```python
from build123d import *

# Parameters (mm, degrees)
SKETCH2_W           = 457.2
SKETCH2_H           = 457.2
BOSS_EXTRUDE3_DEPTH = 4.445
SKETCH3_R           = 3.175
SKETCH3_R_2         = 3.9751
CUT_EXTRUDE1_DEPTH  = 324.31977673
SKETCH4_W           = 457.2
SKETCH4_H           = 457.2
SKETCH4_R           = 3.175
CUT_EXTRUDE2_DEPTH  = 324.31977673


with BuildPart() as part:
    # Sketch2 → Boss-Extrude3 (new body)
    with BuildSketch(Plane.XY):
        Rectangle(SKETCH2_W, SKETCH2_H)
    extrude(amount=BOSS_EXTRUDE3_DEPTH)

    # Sketch3 → Cut-Extrude1 (cut, through all)
    with BuildSketch(Plane(origin=(0, 0, 0), x_dir=(-1, 0, 0), z_dir=(0, 0, -1))):
        with Locations((-138.143199548, 71.871365193)):
            Circle(SKETCH3_R)
        with Locations((-198.809547248, -25.000118004)):
            Circle(SKETCH3_R)
        with Locations((-122.004659563, -96.265887155)):
            Circle(SKETCH3_R)
        with Locations((-26.754659563, -96.265887155)):
            Circle(SKETCH3_R)
        with Locations((-26.754659563, 23.469712845)):
            Circle(SKETCH3_R_2)
    extrude(amount=-CUT_EXTRUDE1_DEPTH, mode=Mode.SUBTRACT)

    # Sketch4 → Cut-Extrude2 (cut, through all)
    # profile 1 of 5: a face of its own
    with BuildSketch(Plane.XY.offset(4.445)):
        Rectangle(SKETCH4_W, SKETCH4_H)
        with Locations((26.754659563, -96.265887155)):
            Circle(SKETCH4_R, mode=Mode.SUBTRACT)
        with BuildLine():
            Line((104.279919091, -89.284764381), (29.57120013, 4.629075933))
            ThreePointArc((29.57120013, 4.629075933), (8.270979184, 28.080142289), (38.089671454, 38.780493538))
            Line((38.089671454, 38.780493538), (119.216168571, 74.032383096))
            ThreePointArc((119.216168571, 74.032383096), (139.225456422, 90.890598092), (157.193199548, 71.871365193))
            ThreePointArc((157.193199548, 71.871365193), (156.629627395, 67.271964637), (154.972256192, 62.944699943))
            Line((154.972256192, 62.944699943), (198.125737804, -5.962394804))
            ThreePointArc((198.125737804, -5.962394804), (212.035958895, -11.290102141), (217.859547248, -25.000118004))
            ThreePointArc((217.859547248, -25.000118004), (210.121888692, -40.327656327), (193.194620104, -43.203828976))
            Line((193.194620104, -43.203828976), (140.576999281, -92.026701216))
            ThreePointArc((140.576999281, -92.026701216), (140.934867851, -94.13288125), (141.054659563, -96.265887155))
            ThreePointArc((141.054659563, -96.265887155), (118.451759762, -114.981639959), (104.279919091, -89.284764381))
        make_face(mode=Mode.SUBTRACT)
    # profile 2 of 5: a face of its own
    with BuildSketch(Plane.XY.offset(4.445)):
        with BuildLine():
            ThreePointArc((127.085491453, 56.359125133), (126.946386449, 56.459231128), (126.808187657, 56.5605845))
            Line((126.808187657, 56.5605845), (55.070704112, 25.388502171))
            Line((55.070704112, 25.388502171), (122.29505865, 6.450632186))
            Line((122.29505865, 6.450632186), (127.085491453, 56.359125133))
        make_face()
    # profile 3 of 5: a face of its own
    with BuildSketch(Plane.XY.offset(4.445)):
        Polygon((144.946705866, 43.06176458), (140.928758156, 1.201305791), (177.638536292, -9.140258814), align=None)
    # profile 4 of 5: a face of its own
    with BuildSketch(Plane.XY.offset(4.445)):
        Polygon((179.886249099, -29.564951481), (139.079100318, -18.069110674), (133.87810257, -72.255020413), align=None)
    # profile 5 of 5: a face of its own
    with BuildSketch(Plane.XY.offset(4.445)):
        Polygon((120.445400812, -12.81978428), (52.587094953, 6.296677047), (114.776579601, -71.879651121), align=None)
    extrude(amount=-CUT_EXTRUDE2_DEPTH, mode=Mode.SUBTRACT)


solid = part.part
```
Verification items for the finished model (mm, model axes). A direction names the side the tool comes from. Round coordinates to 2 decimals unless told otherwise and drop trailing zeros. Write each loop counter-clockwise with the first axis right and the second up, starting at its lowest first coordinate (ties: lowest second). Pieces come first, ordered by that corner, then holes. Notation, with made-up numbers: (44.25, 86) -> (103.25, 86) arc R35 cw to (103.25, 122) -> close; hole circle Ø8 at (20.25, 46.5). An arc over 180 degrees is marked (long way). Write each question's results on one line, items separated by ' | '. Start each with the question number.
1. Cross-section at D-D (z = 1.1). Count the separate pieces of the cut face and the enclosed holes in it, then the cut area to 3 significant figures.
2. Cross-section at C-C (x = 161). Enter the section's corners in (y, z) (3 decimals), then the cut area to 3 significant figures.
3. Cross-section at B-B (x = 26). Enter the section's corners in (y, z) (3 decimals), then the cut area to 3 significant figures.
4. Material ranges on probe 1 along Y at (x, z) = (93.5, 3.05); probe 2 along X at (y, z) = (-68.5, 4.3); probe 3 along Y at (x, z) = (27, 3.95), recorded low to high. Write a range as from..to.
5. Set-up check for faces 1 (the flat face through (156.56, -51.21, 2.25)), 2 (the flat face through (135, -11, 4.445)): record each of +Z, -Z, +X, -X, +Y, -Y from which the full face is reachable in a straight line by a thin tool's end or side.
6. Cross-section at A-A (y = -56). Enter the section's corners in (x, z) (3 decimals).
7. Depth check by flat-ended pin: P1, Ø2, axis at y = 61, z = 2.5, coming from the +X side; P2, Ø7, axis at x = 26.75, y = 23.47, coming from the -Z side; P3, Ø1.5, axis at x = 147, z = 3.5, coming from the +Y side; P4, Ø2, axis at x = 36.5, z = 3.5, coming from the -Y side. Enter the tip coordinate at first touch or a pass-through.
Solutions:
1) separate pieces: 1 | enclosed holes: 8 | area: 15,700 mm2
2) outline: (-73.077, 0) -> (-47.089, 0) -> (-47.089, 4.445) -> (-73.077, 4.445) -> close; (-24.244, 0) -> (-4.453, 0) -> (-4.453, 4.445) -> (-24.244, 4.445) -> close; (17.428, 0) -> (53.32, 0) -> (53.32, 4.445) -> (17.428, 4.445) -> close | area: 363 mm2
3) outline: (4.435, 0) -> (19.567, 0) -> (19.567, 4.445) -> (4.435, 4.445) -> close; (27.373, 0) -> (42.505, 0) -> (42.505, 4.445) -> (27.373, 4.445) -> close | area: 135 mm2
4) probe 1: y = -75.73..-45.13, -5.23..14.56, 42.09..62.86 | probe 2: x = 87.75..112.09, 115.1..134.24, 137.92..165.93 | probe 3: y = 4.42..19.5, 27.44..42.52
5) face 1: +Z, -Z | face 2: +Z, +X, -X, +Y, -Y
6) outline: (77.802, 0) -> (102.144, 0) -> (102.144, 4.445) -> (77.802, 4.445) -> close; (116.301, 0) -> (135.438, 0) -> (135.438, 4.445) -> (116.301, 4.445) -> close; (151.397, 0) -> (179.404, 0) -> (179.404, 4.445) -> (151.397, 4.445) -> close
7) P1: stops at x = 156.82 | P2: passes through | P3: stops at y = 89.11 | P4: stops at y = -5.34
